Autodesk Inventor part; units mm, degrees
ref_plane "Work Plane5" through (17.5, 0, 0) normal (1, 0, 0) x (0, 1, 0)
ref_plane "Work Plane6" through (0, 30, 0) normal (0, -1, 0) x (1, 0, 0)
ref_plane "Work Plane7" through (0, 0, -17.5) normal (0, 0, 1) x (1, 0, 0)
sketch "Sketch1" plane through (0, 0, 0) normal (0, 1, 0) x (-1, 0, 0)
  line L0 (0, -24.5) -> (0, 24.5) construction
  line L1 (-24.5, 0) -> (24.5, 0) construction
  circle A0 centre (0, 0) radius 17.5
  circle A1 centre (0, 0) radius 15
  dimension "d0" = 35
  dimension "d1" = 30
extrude "Extrusion1" add sketch "Sketch1" along normal blind 60
ref_plane "Work Plane5" through (17.5, 0, 0) normal (1, 0, 0) x (0, 1, 0)
ref_plane "Work Plane6" through (0, 30, 0) normal (0, -1, 0) x (1, 0, 0)
sketch "Sketch7" plane through (0, 30, 0) normal (0, -1, 0) x (1, 0, 0)
  circle A0 centre (0, 0) radius 15 construction
  line L0 (0, 24.5) -> (0, -24.5) construction
  line L1 (-34.4, 0) -> (83.9, 0) construction
  arc A1 (61.225, -6.892) -> (61.225, 6.892) centre (60, 0) ccw
  line L2 (3.0625, -17.2299) -> (61.225, -6.892)
  line L3 (3.0625, 17.2299) -> (61.225, 6.892)
  arc A2 (3.0625, -17.2299) -> (3.0625, 17.2299) centre (0, 0) ccw
  circle A3 centre (60, 0) radius 4
  dimension "d35" = 14
  dimension "d36" = 60
  dimension "d37" = 8
extrude "Extrusion5" add sketch "Sketch7" along normal mid plane 3
ref_plane "Work Plane7" through (0, 0, -17.5) normal (0, 0, 1) x (1, 0, 0)
sketch "Sketch8" plane through (0, 0, -17.5) normal (0, 0, 1) x (1, 0, 0)
  circle A0 centre (0, 25) radius 6
  circle A1 centre (0, 25) radius 8.5
  point P0 (0, 0)
extrude "Extrusion6" add sketch "Sketch8" against normal blind 55 contours A0 | A1
extrude "Extrusion7" add sketch "Sketch8" against normal blind 70 contours A0
extrude "Extrusion8" add sketch "Sketch8" along normal up to next contours A0 | A1
thread "Thread2"
equation "\"d23\" = 55deg"
equation "\"Sketch4_Pitch\" = 1.75"
properties part number "steering_kingpin_right" material "Steel, Mild"
For this review, take the finished solid that the model builds, in its own axes (mm). A direction names the side the tool comes from. Round coordinates to 2 decimals unless told otherwise and drop trailing zeros. Write each loop counter-clockwise with the first axis right and the second up, starting at its lowest first coordinate (ties: lowest second). Pieces come first, ordered by that corner, then holes. Notation, with made-up numbers: (-36, -9.75) - (-30, -9.75) arc R11 ccw to (-30, 1.25) - close; hole circle Ø9 at (-1.75, 26.5). An arc over 180 degrees is marked (long way). Answer as a JSON object with one key per item and string values.
1. For pin 1 Ø18 at (x, z) = (0, 0) entering from +Y; pin 2 Ø8 at (y, z) = (18.5, -55) entering from +X; pin 3 Ø3 at (x, y) = (-2.5, 36) entering from -Z, all flat-tipped, find the tip position at first contact; note any pin that passes through.
Response values:
{"pin 1": "passes through", "pin 2": "stops at x = 8.12", "pin 3": "stops at z = -17.47"}
2. To check wall thickness, follow line 1 along Z through (x, y) = (0, 36.5); line 2 along Z through (x, y) = (60, 29); line 3 along X through (y, z) = (54.5, -8). State the ranges of each line that lie inside material, in increasing order.
Response values:
{"line 1": "z = -17.5 to -15, 15 to 17.5", "line 2": "z = -7.11 to -4, 4 to 7.11", "line 3": "x = -15.56 to -12.69, 12.69 to 15.56"}
3. We need section B-B on x = 0. Give the boundary of the cut face in (y, z), then the cut area to 4 significant figures.
Response values:
{"outline": "(0, -17.5) - (16.5, -17.5) - (16.5, -72.5) - (19, -72.5) - (19, -87.5) - (31, -87.5) - (31, -72.5) - (33.5, -72.5) - (33.5, -17.5) - (60, -17.5) - (60, -15) - (0, -15) - close; (0, 15) - (60, 15) - (60, 17.5) - (0, 17.5) - close", "area": "1,415 mm2"}
4. Draft analysis for pull direction X (two halves, no side actions). For faces 4 (the face through (63.815, 30.021, -1.201)), 5 (the face through (31.76, 30.02, 12.13)), 6 (the face through (-1.301, 19.143, -79.895)), 7 (the face through (-6, 23, -72.5)), state which applies: +X half, -X half, draft (parallel to the pull), parting line (faces both ways), or undercut.
Response values:
{"face 4": "undercut", "face 5": "+X half", "face 6": "parting line", "face 7": "draft"}
5. We need section D-D on x = 60. Give the boundary of the cut face in (y, z), then the cut area to 3 significant figures.
Response values:
{"outline": "(28.5, -7.11) - (31.5, -7.11) - (31.5, -4) - (28.5, -4) - close; (28.5, 4) - (31.5, 4) - (31.5, 7.11) - (28.5, 7.11) - close", "area": "18.7 mm2"}
6. We need section A-A on z = 0. Give the boundary of the cut face in (x, y), then the cut area to 4 significant figures.
Response values:
{"outline": "(-17.5, 0) - (-15, 0) - (-15, 60) - (-17.5, 60) - close; (15, 0) - (17.5, 0) - (17.5, 28.5) - (56, 28.5) - (56, 31.5) - (17.5, 31.5) - (17.5, 60) - (15, 60) - close; (64, 28.5) - (67, 28.5) - (67, 31.5) - (64, 31.5) - close", "area": "424.5 mm2"}
7. We need section C-C on y = 25. Give the boundary of the cut face in (x, z).
Response values:
{"outline": "(-8.5, -72.5) - (-6, -72.5) - (-6, -87.5) - (6, -87.5) - (6, -72.5) - (8.5, -72.5) - (8.5, -15.3) arc R17.5 ccw (long way) to (-8.5, -15.3) - close; hole circle Ø30 at (0, 0)"}
8. Tool access review of faces 1 (the face through (-16.166, 29.58, 6.703)), 2 (the face through (4, 17.5, -44.3)), 3 (the face through (14.985, 29.58, -0.66)): name each direction out of +Z, -Z, +X, -X, +Y, -Y from which nothing blocks a thin tool from reaching the whole face with its end or side.
Response values:
{"face 1": "none", "face 2": "-Z", "face 3": "+Y, -Y"}
